Here's how the part is built. I have some questions about the finished solid (model axes, mm). A direction names the side the tool comes from. Coordinates: 2 decimals unless noted, no trailing zeros. Loops run counter-clockwise (first coordinate to the right, second up) from the corner with the lowest first, then second, coordinate; pieces in that order, holes last.
```python
from build123d import *

# Parameters (mm, degrees)
BOSS_EXTRUDE1_DEPTH  = 21
SKETCH2_R            = 1.825
CUT_EXTRUDE1_DEPTH   = 4
SKETCH3_W            = 7.5
SKETCH3_H            = 11.75
CUT_EXTRUDE2_DEPTH   = 13
FILLET1_R            = 4
SKETCH5_R            = 1.825
CUT_EXTRUDE3_DEPTH   = 41.522370365
FILLET1_OF_MIRROR1_R = 4
CUT_EXTRUDE5_DEPTH   = 44.75
FILLET2_R            = 1
FILLET3_R            = 9
FILLET4_R            = 3
SKETCH11_R           = 3.75
CUT_EXTRUDE6_DEPTH   = 68.788734315


with BuildPart() as part:
    # Sketch1 → Boss-Extrude1 (new body)
    with BuildSketch(Plane(origin=(0, 0, 0), x_dir=(1, 0, 0), z_dir=(0, 1, 0))):
        Polygon((-24.5, 0), (-24.5, 12.75), (0, 12.75), (0, 15.75), (-35, 15.75), (-35, 0), align=None)
    boss_extrude1 = extrude(amount=BOSS_EXTRUDE1_DEPTH)

    # Sketch2 → Cut-Extrude1 (cut)
    with BuildSketch(Plane.XY):
        with Locations((-31.25, 7)):
            Circle(SKETCH2_R)
    cut_extrude1 = extrude(amount=-CUT_EXTRUDE1_DEPTH, mode=Mode.SUBTRACT)

    # Sketch3 → Cut-Extrude2 (cut)
    with BuildSketch(Plane.XZ):
        with Locations((-31.25, -9.875)):
            Rectangle(SKETCH3_W, SKETCH3_H)
    cut_extrude2 = extrude(amount=-CUT_EXTRUDE2_DEPTH, mode=Mode.SUBTRACT)

    # Fillet1
    fillet1_edges = [part.edges().sort_by_distance(p)[0] for p in [
        (-35, 17, -15.75),
    ]]
    fillet(fillet1_edges, radius=FILLET1_R)

    # Sketch5 → Cut-Extrude3 (cut, through all)
    with BuildSketch(Plane.XZ.offset(-13)):
        with Locations(Location((-31, -11.75, 0), (0, 0, 270))):
            Circle(SKETCH5_R)
    cut_extrude3 = extrude(amount=-CUT_EXTRUDE3_DEPTH, mode=Mode.SUBTRACT)

    # Mirror1: Boss-Extrude1, Cut-Extrude1, Cut-Extrude2, Cut-Extrude3 across plane
    add(boss_extrude1.mirror(Plane(origin=(0, 21, 0), x_dir=(0, 0, 1), z_dir=(-1, 0, 0))))
    add(cut_extrude1.mirror(Plane(origin=(0, 21, 0), x_dir=(0, 0, 1), z_dir=(-1, 0, 0))), mode=Mode.SUBTRACT)
    add(cut_extrude2.mirror(Plane(origin=(0, 21, 0), x_dir=(0, 0, 1), z_dir=(-1, 0, 0))), mode=Mode.SUBTRACT)
    add(cut_extrude3.mirror(Plane(origin=(0, 21, 0), x_dir=(0, 0, 1), z_dir=(-1, 0, 0))), mode=Mode.SUBTRACT)

    # Fillet1 of Mirror1
    fillet1_of_mirror1_edges = [part.edges().sort_by_distance(p)[0] for p in [
        (35, 17, -15.75),
    ]]
    fillet(fillet1_of_mirror1_edges, radius=FILLET1_OF_MIRROR1_R)

    # Sketch10 → Cut-Extrude5 (cut, through all)
    with BuildSketch(Plane(origin=(0, 0, -15.75), x_dir=(-1, 0, 0), z_dir=(0, 0, -1))):
        Polygon((-24, 3), (-3.793861182, 3), (-24, 16.969897852), align=None)
        Polygon((-21.093861182, 18), (-1.25, 18), (-1.25, 4.280569672), align=None)
        Polygon((24, 3), (24, 16.969897852), (3.793861182, 3), align=None)
        Polygon((21.093861182, 18), (1.25, 4.280569672), (1.25, 18), align=None)
    extrude(amount=-CUT_EXTRUDE5_DEPTH, mode=Mode.SUBTRACT)

    # Fillet2
    fillet2_edges = [part.edges().sort_by_distance(p)[0] for p in [
        (-24, 3, -14.25),
        (-3.793861182, 3, -14.25),
        (-24, 16.969897852, -14.25),
        (24, 3, -14.25),
        (24, 16.969897852, -14.25),
        (3.793861182, 3, -14.25),
        (-1.25, 18, -14.25),
        (-21.093861182, 18, -14.25),
        (-1.25, 4.280569672, -14.25),
        (1.25, 4.280569672, -14.25),
        (21.093861182, 18, -14.25),
        (1.25, 18, -14.25),
    ]]
    fillet(fillet2_edges, radius=FILLET2_R)

    # Fillet3
    fillet3_edges = [part.edges().sort_by_distance(p)[0] for p in [
        (-29.75, 21, 0),
        (29.75, 21, 0),
    ]]
    fillet(fillet3_edges, radius=FILLET3_R)

    # Fillet4
    fillet4_edges = [part.edges().sort_by_distance(p)[0] for p in [
        (-27.5, 6.5, -15.75),
        (27.5, 6.5, -15.75),
    ]]
    fillet(fillet4_edges, radius=FILLET4_R)

    # Sketch11 → Cut-Extrude6 (cut, through all)
    with BuildSketch(Plane(origin=(27.5, 0, 0), x_dir=(0, 0, -1), z_dir=(1, 0, 0))):
        with Locations((8.375, 6.5)):
            Circle(SKETCH11_R)
    extrude(amount=-CUT_EXTRUDE6_DEPTH, mode=Mode.SUBTRACT)


solid = part.part
```
1. I want a section at B-B (x = -5). Please give me the cut outline in (y, z), then the cut area to 3 significant figures.
2. I need wall thicknesses on line 1 along X through (y, z) = (18.5, -11.75) (3 decimals); line 2 along Y through (x, z) = (-31.25, -3.2) (3 decimals); line 3 along X through (y, z) = (4.5, -15). Which ranges of each line are inside material? Lowest first, please.
3. On a 3-axis mill with a long thin cutter (end or side, diameter ignored), from which of +Z, -Z, +X, -X, +Y, -Y can I reach the whole of each face in a straight line? I mean faces 1 (the flat face through (0, 10, -12.75)), 2 (the flat face through (0, 13, -15.75)), 3 (the cylindrical face through (26.6, 6.59, -14.89)), 4 (the flat face through (-15, 3, -14)), 5 (the cylindrical face through (26.02, 4.22, -5.4)). Say none if no direction works.
4. I want a section at A-A (z = -7.75). Please give me the cut outline in (x, y).
5. For pin 1 (3 mm diameter, centred on x = -32, z = -12.5, fed in from -Y); pin 2 (7 mm diameter, centred on y = 6.5, z = -8.375, fed in from -X); pin 3 (1 mm diameter, centred on y = 2.5, z = -13, fed in from -X); pin 4 (12 mm diameter, centred on x = -15, y = 6, fed in from +Z), each with a flat end and sliding along its axis, tell me the tip position at first contact or that it passes through.
6. We'd pull the mould along Y, two halves only. Please class faces 6 (the cylindrical face through (-6, 4, -14)), 7 (the cylindrical face through (29.676, 18.434, -2.706)), 8 (the cylindrical face through (-33.859, 17.056, -14.547)): +Y half, -Y half, draft (parallel to the pull), parting line (faces both ways), or undercut.
7. I want a section at C-C (z = -11). Please give me the cut outline in (x, y).
Response values:
1. outline: (0, -15.75) - (6.87, -15.75) - (6.87, -12.75) - (0, -12.75) - close; (18, -15.75) - (21, -15.75) - (21, -12.75) - (18, -12.75) - close
1. area: 29.6 mm2
2. line 1: x = -35 to -32.825, -29.175 to -24.5, 24.5 to 29.175, 32.825 to 35
2. line 2: y = 0 to 5.175, 8.825 to 18.882
2. line 3: x = -26.48 to -24, -6.13 to 6.13, 24 to 26.48
3. face 1: +Z, +Y, -Y
3. face 2: -Z, +X, -X, +Y, -Y
3. face 3: -Z, +X, -Y
3. face 4: +Z, -Z
3. face 5: +X, -X
4. outline: (-35, 13) - (-27.5, 13) - (-27.5, 10.2) - (-24.5, 10.2) - (-24.5, 20.91) - (-35, 20.91) - close; (-27.5, 0) - (-24.5, 0) - (-24.5, 2.8) - (-27.5, 2.8) - close; (24.5, 0) - (27.5, 0) - (27.5, 2.8) - (24.5, 2.8) - close; (24.5, 10.2) - (27.5, 10.2) - (27.5, 13) - (35, 13) - (35, 20.91) - (24.5, 20.91) - close
5. pin 1: stops at y = 13
5. pin 2: passes through
5. pin 3: stops at x = -27.5
5. pin 4: stops at z = -12.75
6. face 6: undercut
6. face 7: +Y half
6. face 8: draft
7. outline: (-35, 13) - (-32.66, 13) - (-32.66, 21) - (-35, 21) - close; (-29.34, 13) - (-27.5, 13) - (-27.5, 9.18) - (-24.5, 9.18) - (-24.5, 21) - (-29.34, 21) - close; (-27.5, 0) - (-24.5, 0) - (-24.5, 3.82) - (-27.5, 3.82) - close; (24.5, 0) - (27.5, 0) - (27.5, 3.82) - (24.5, 3.82) - close; (24.5, 9.18) - (27.5, 9.18) - (27.5, 13) - (29.34, 13) - (29.34, 21) - (24.5, 21) - close; (32.66, 13) - (35, 13) - (35, 21) - (32.66, 21) - close
